Design review of the part built by this model. Coordinates are the model's own, in mm. Coordinates: 2 decimals unless noted, no trailing zeros. Loops run counter-clockwise (first coordinate to the right, second up) from the corner with the lowest first, then second, coordinate; pieces in that order, holes last.
Q1. Wall thickness on probe 1 along Z at (x, y) = (0, 1.4) (3 decimals); probe 2 along Z at (x, y) = (32.5, 2.9); probe 3 along Z at (x, y) = (-48.5, 4.15): over which ranges is each line inside the solid? List them lowest first.
Q2. Add section D-D on x = -28.5. Give the boundary of the cut face in (y, z).
Q3. Add section B-B on y = 0.85. Give the number of separate pieces and of enclosed holes in the cut face, and give its area (3 significant figures).
Q4. Add section A-A on x = 0. Give the boundary of the cut face in (y, z) (1 decimal), and give its area (3 significant figures).
Q5. For P1, Ø1, axis at y = 3.5, z = 1, coming from the +X side; P2, Ø0.9, axis at x = 33.5, y = 3.5, coming from the -Z side; P3, Ø1.9, axis at x = 65.5, y = 2.5, coming from the +Z side; P4, Ø18, axis at x = 0, z = 0, coming from the +Y side, all flat-tipped, find the tip position at first contact; note any pin that passes through.
Q6. Add section C-C on z = 66.5. Give the boundary of the cut face in (x, y).
```python
from build123d import *

# Parameters (mm, degrees)
SKETCH1_R           = 80
SKETCH1_R_2         = 7.875
BOSS_EXTRUDE1_DEPTH = 4.7625
CUT_EXTRUDE1_DEPTH  = 5.7625
BOSS_EXTRUDE2_DEPTH = 4.7625
CUT_EXTRUDE2_DEPTH  = 5.7625
CUT_EXTRUDE5_DEPTH  = 5.7625
FILLET1_R           = 2
SKETCH8_W           = 3
SKETCH8_H           = 5.5
CUT_EXTRUDE6_DEPTH  = 5.7625


with BuildPart() as part:
    # Sketch1 → Boss-Extrude1 (new body)
    with BuildSketch(Plane(origin=(0, 0, 0), x_dir=(1, 0, 0), z_dir=(0, 1, 0))):
        Circle(SKETCH1_R)
        Circle(SKETCH1_R_2, mode=Mode.SUBTRACT)
    extrude(amount=BOSS_EXTRUDE1_DEPTH)

    # Sketch2 → Cut-Extrude1 (cut, through all)
    with BuildSketch(Plane(origin=(0, 4.7625, 0), x_dir=(1, 0, 0), z_dir=(0, 1, 0))):
        with BuildLine():
            Line((34.2, 0), (70.8, 0))
            Line((70.8, 0), (70.8, 3))
            ThreePointArc((70.8, 3), (70.653553391, 3.353553391), (70.3, 3.5))
            Line((70.3, 3.5), (67.3, 3.5))
            ThreePointArc((67.3, 3.5), (66.946446609, 3.353553391), (66.8, 3))
            Line((66.8, 3), (66.8, 2))
            ThreePointArc((66.8, 2), (66.653553391, 1.646446609), (66.3, 1.5))
            Line((66.3, 1.5), (64.55, 1.5))
            ThreePointArc((64.55, 1.5), (64.196446609, 1.646446609), (64.05, 2))
            Line((64.05, 2), (64.05, 3))
            ThreePointArc((64.05, 3), (63.903553391, 3.353553391), (63.55, 3.5))
            Line((63.55, 3.5), (52.95, 3.5))
            Line((52.95, 3.5), (39.164998359, 2.532631464))
            ThreePointArc((39.164998359, 2.532631464), (38.834280968, 2.374812024), (38.7, 2.033858083))
            Line((38.7, 2.033858083), (38.7, 2))
            ThreePointArc((38.7, 2), (38.553553391, 1.646446609), (38.2, 1.5))
            Line((38.2, 1.5), (34.7, 1.5))
            ThreePointArc((34.7, 1.5), (34.346446609, 1.353553391), (34.2, 1))
            Line((34.2, 1), (34.2, 0))
        make_face()
    extrude(amount=-CUT_EXTRUDE1_DEPTH, mode=Mode.SUBTRACT)

    # Sketch4 → Boss-Extrude2 (add)
    with BuildSketch(Plane(origin=(0, 4.7625, 0), x_dir=(1, 0, 0), z_dir=(0, 1, 0))):
        Polygon((-88, 32.5), (-60, 37.43715546), (-60, -37.43715546), (-88, -32.5), (-88, -16.5), (-71.5, 0), (-88, 16.5), align=None)
        with BuildLine():
            Line((78.751819834, 14.076607291), (91.414213562, 1.414213562))
            ThreePointArc((91.414213562, 1.414213562), (92, 0), (91.414213562, -1.414213562))
            Line((91.414213562, -1.414213562), (78.751819834, -14.076607291))
            Line((78.751819834, -14.076607291), (78.751819834, 14.076607291))
        make_face()
    extrude(amount=-BOSS_EXTRUDE2_DEPTH)

    # Sketch3 → Cut-Extrude2 (cut, through all)
    with BuildSketch(Plane(origin=(0, 4.7625, 0), x_dir=(1, 0, 0), z_dir=(0, 1, 0))):
        with BuildLine():
            Line((75.187234449, 9.826135427), (74.687234449, 9.826135427))
            ThreePointArc((74.687234449, 9.826135427), (74.062234449, 9.201135427), (74.687234449, 8.576135427))
            Line((74.687234449, 8.576135427), (84.252291698, 8.576135427))
            Line((84.252291698, 8.576135427), (78.751819834, 14.076607291))
            ThreePointArc((78.751819834, 14.076607291), (78.803418829, 13.784817039), (78.853936691, 13.492837669))
            Line((78.853936691, 13.492837669), (75.187234449, 9.826135427))
        make_face()
    extrude(amount=-CUT_EXTRUDE2_DEPTH, mode=Mode.SUBTRACT)

    # Sketch7 → Cut-Extrude5 (cut, through all)
    with BuildSketch(Plane(origin=(0, 4.7625, 0), x_dir=(1, 0, 0), z_dir=(0, 1, 0))):
        with BuildLine():
            Line((-88, 22), (-77.424613279, 20.13527399))
            ThreePointArc((-77.424613279, 20.13527399), (-78.737936574, 14.154057514), (-79.589907619, 8.089907619))
            Line((-79.589907619, 8.089907619), (-88, 16.5))
            Line((-88, 16.5), (-88, 22))
        make_face()
    extrude(amount=-CUT_EXTRUDE5_DEPTH, mode=Mode.SUBTRACT)

    # Fillet1
    fillet1_edges = [part.edges().sort_by_distance(p)[0] for p in [
        (-88, 2.38125, -22),
        (-71.75940266, 2.38125, 35.363655494),
        (-71.75940266, 2.38125, -35.363655494),
        (-88, 2.38125, -32.5),
        (-88, 2.38125, 16.5),
        (-88, 2.38125, 32.5),
    ]]
    fillet(fillet1_edges, radius=FILLET1_R)

    # Sketch8 → Cut-Extrude6 (cut, through all)
    with BuildSketch(Plane(origin=(0, 4.7625, 0), x_dir=(1, 0, 0), z_dir=(0, 1, 0))):
        with Locations((33.625, 0.75)):
            Rectangle(SKETCH8_W, SKETCH8_H)
        with Locations((71.375, 0.75)):
            Rectangle(SKETCH8_W, SKETCH8_H)
    extrude(amount=-CUT_EXTRUDE6_DEPTH, mode=Mode.SUBTRACT)


solid = part.part
```
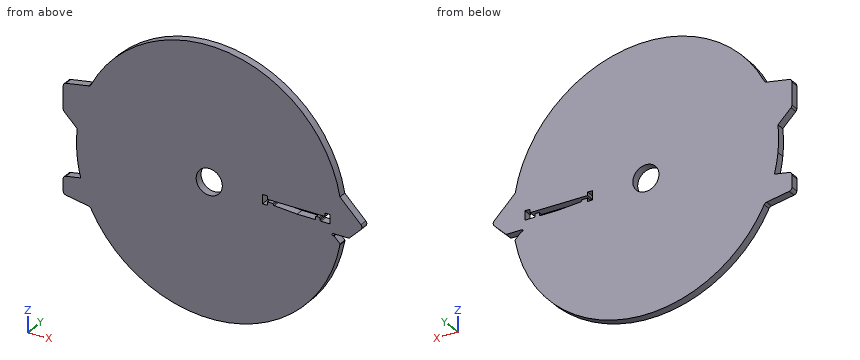
Entries:
1. probe 1: z = -80 to -7.875, 7.875 to 80
1. probe 2: z = -73.1 to -3.5, 2 to 73.1
1. probe 3: z = -63.62 to 63.62
2. outline: (0, -74.75) - (4.76, -74.75) - (4.76, 74.75) - (0, 74.75) - close
3. separate pieces: 1
3. enclosed holes: 2
3. area: 20,300 mm2
4. outline: (0, -80) - (4.8, -80) - (4.8, -7.9) - (0, -7.9) - close; (0, 7.9) - (4.8, 7.9) - (4.8, 80) - (0, 80) - close
4. area: 687 mm2
5. P1: stops at x = 91.94
5. P2: stops at z = -72.85
5. P3: stops at z = 47.26
5. P4: stops at y = 4.76
6. outline: (-44.47, 0) - (44.47, 0) - (44.47, 4.76) - (-44.47, 4.76) - close
